from build123d import *

# Parameters (mm, degrees)
BOSS_EXTRU_1_DEPTH = 3
CHANFREIN1_SIZE    = 1


with BuildPart() as part:
    # Esquisse1 → Boss.-Extru.1 (new body)
    with BuildSketch(Plane(origin=(0, 0, 0), x_dir=(1, 0, 0), z_dir=(0, 1, 0))):
        with BuildLine():
            Line((-3.5, 3.8), (3.5, 3.8))
            ThreePointArc((3.5, 3.8), (7.3, 0), (3.5, -3.8))
            Line((3.5, -3.8), (-3.5, -3.8))
            ThreePointArc((-3.5, -3.8), (-7.3, 0), (-3.5, 3.8))
        make_face()
    extrude(amount=BOSS_EXTRU_1_DEPTH)

    # Chanfrein1
    chanfrein1_edges = [part.edges().sort_by_distance(p)[0] for p in [
        (7.3, 3, 0),
        (0, 3, -3.8),
        (-7.3, 3, 0),
        (0, 3, 3.8),
    ]]
    chamfer(chanfrein1_edges, length=CHANFREIN1_SIZE)


solid = part.part
Input: part model. Units: mm. Frame: model coordinates. Coordinates: 2 decimals unless noted, no trailing zeros. Order: outer loops, then holes, each group sorted by start corner. A loop starts at its lowest first (then second) coordinate and runs counter-clockwise, first axis right, second up.
1. Ray query, line 1 along Y through (x, z) = (-3.25, -3); line 2 along Z through (x, y) = (2.75, 2.95); line 3 along Z through (x, y) = (6.25, 2.2). Return the intervals inside material, ascending.
Checked values:
line 1: y = 0 to 2.8
line 2: z = -2.85 to 2.85
line 3: z = -2.32 to 2.32
2. Cut plane B-B, the plane z = 0. Return loops of the section in (x, y).
Checked values:
outline: (-7.3, 0) - (7.3, 0) - (7.3, 2) - (6.3, 3) - (-6.3, 3) - (-7.3, 2) - close
3. Contact query for flat-ended pins moving along their axis: P1, Ø1.5, axis at x = -5.5, y = 0.5, coming from the -Z side; P2, Ø1, axis at y = 1, z = 2, coming from the -X side. Output: stop coordinate, or through.
Checked values:
P1: stops at z = -3.59
P2: stops at x = -6.99
4. Cut plane A-A, the plane x = 3. Return loops of the section in (y, z), plus the area to 3 significant figures.
Checked values:
outline: (0, -3.8) - (2, -3.8) - (3, -2.8) - (3, 2.8) - (2, 3.8) - (0, 3.8) - close
area: 21.8 mm2
5. Cut plane C-C, the plane y = 1.3. Return loops of the section in (x, z), plus the area to 3 significant figures.
Checked values:
outline: (-3.5, -3.8) - (3.5, -3.8) arc R3.8 ccw to (3.5, 3.8) - (-3.5, 3.8) arc R3.8 ccw to start
area: 98.6 mm2
